Source: CAD feature listing. Evaluate the final solid. Frame: model axes, mm. Face numbers are marked on the shaded views. Round coordinates to 2 decimals unless told otherwise and drop trailing zeros. Write each loop counter-clockwise with the first axis right and the second up, starting at its lowest first coordinate (ties: lowest second). Pieces come first, ordered by that corner, then holes. Notation, with made-up numbers: (8, -34) - (62, -34) arc R12 cw to (62, -26) - close; hole circle Ø1 at (15, -31.75). An arc over 180 degrees is marked (long way). Write item = value, one per line. Start each with the question number.
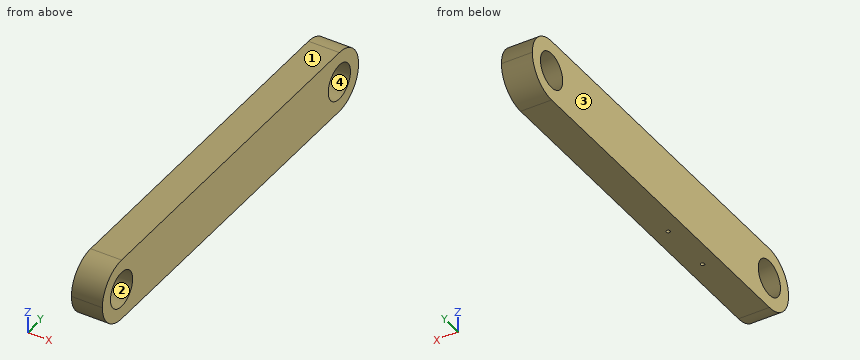
```python
from build123d import *

# Parameters (mm, degrees)
F0_W     = 19.05
F0_H     = 38.1
F1_DEPTH = 254
F3_D     = 22
F4_R     = 19.04999
F5_R     = 1.190625
F6_DEPTH = 12.7


# Not quite as in the source:
# - a fillet or chamfer is up to 0.001 mm smaller than in the source, because OpenCascade refuses the exact size


with BuildPart() as f1:
    # F0 (on Front) → F1 (new body)
    with BuildSketch(Plane.XZ):
        Rectangle(F0_W, F0_H)
    extrude(amount=-F1_DEPTH)

    # F3 (through all)
    with Locations(Plane.YZ.offset(9.525)):
        with Locations((19.05, 0), (234.95, 0)):
            Hole(F3_D / 2)

    # F4 (radius 19.05 in the source; OpenCascade refuses exactly that, so slightly less here)
    f4_edges = [f1.edges().sort_by_distance(p)[0] for p in [
        (0, 0, 19.05),
        (0, 0, -19.05),
        (0, 254, 19.05),
        (0, 254, -19.05),
    ]]
    fillet(f4_edges, radius=F4_R)

    # F5 (on face) → F6 (cut)
    with BuildSketch(Plane(origin=(0, 0, -19.05), x_dir=(1, 0, 0), z_dir=(0, 0, -1))):
        with Locations((0, -103.98125)):
            Circle(F5_R)
        with Locations((0, -69.85)):
            Circle(F5_R)
    extrude(amount=-F6_DEPTH, mode=Mode.SUBTRACT)


solid = f1.part
```
(1) Section A-A (x = -3.5). Count the separate pieces of the cut face and the enclosed holes in it, plus the area to 3 significant figures.
(2) Section B-B (z = 6). Return the cut outline in (x, y) (3 decimals).
(3) Ray query, L1, parallel to Z at x = 3.5, y = 234.95; L2, parallel to Y at x = -6, z = 7.5; L3, parallel to Y at x = 4, z = 6.5. Return the intervals inside material, ascending. Write a range as from..to.
(4) Pull-direction query (Z, two-part tool) for the marked faces 1, 2, 3 and 4; classes: +Z half, -Z half, draft (parallel to the pull), parting line (faces both ways), or undercut.
(5) Contact query for flat-ended pins moving along their axis: P1, Ø0.7, axis at x = 0, y = 104.5, coming from the -Z side; P2, Ø1.9, axis at x = 0.5, y = 70, coming from the -Z side. Output: stop coordinate, or through.
Solution:
q1.separate_pieces = 1
q1.enclosed_holes = 2
q1.area = 8,610 mm^2
q2.outline = (-9.525, 0.97) - (9.525, 0.97) - (9.525, 9.83) - (-9.525, 9.83) - close; (-9.525, 28.27) - (9.525, 28.27) - (9.525, 225.73) - (-9.525, 225.73) - close; (-9.525, 244.17) - (9.525, 244.17) - (9.525, 253.03) - (-9.525, 253.03) - close
q3.L1 = -19.05..-11, 11..19.05
q3.L2 = 1.54..11, 27.1..226.9, 243..252.46
q3.L3 = 1.14..10.18, 27.92..226.08, 243.82..252.86
q4.face_1 = +Z half
q4.face_2 = undercut
q4.face_3 = draft
q4.face_4 = undercut
q5.P1 = -6.35
q5.P2 = -19.05
